Design review of the part built by this model. Coordinates are the model's own, in mm. Face numbers are marked on the shaded views. A direction names the side the tool comes from. Give positions to 0.01 mm unless a question says otherwise; leave off trailing zeros. Loops run counter-clockwise (first coordinate to the right, second up) from the corner with the lowest first, then second, coordinate; pieces in that order, holes last. Notation, with made-up numbers: (-9, -12.75) -> (18, -12.75) arc R25 cw to (18, 17.25) -> close; hole circle Ø6 at (47.5, 20). An arc over 180 degrees is marked (long way). Answer in a Markdown table with one row per item. Add a question column.
(1) Consider section A-A on y = 15. Write out the cut boundary in (x, z), then the cut area to 3 significant figures.
(2) For the marked faces 5, 6, 7, 8 and 9, list the 3-axis set-ups (+Z, -Z, +X, -X, +Y, -Y) from which the entire face can be reached by the end or side of a thin tool; tool diameter is ignored.
(3) For pin 1 (3.5 mm diameter, centred on x = 0, y = 49, fed in from -Z); pin 2 (0.5 mm diameter, centred on y = 49, z = 0.5, fed in from -X); pin 3 (2 mm diameter, centred on x = -4.5, z = -6.5, fed in from +Y); pin 4 (6 mm diameter, centred on x = 0.5, z = -0.5, fed in from -Y), all flat-tipped, find the tip position at first contact; note any pin that passes through.
(4) For line 1 (Y direction, x = 0, z = -0.1); line 2 (Y direction, x = 0.75, z = 3.75); line 3 (Y direction, x = 6.75, z = 4.5), list the stretches that pass through material, from the lowest coordinate up.
(5) Draft analysis for pull direction Y (two halves, no side actions). For the marked faces 1, 2, 3 and 4, state which applies: +Y half, -Y half, draft (parallel to the pull), parting line (faces both ways), or undercut.
(6) Consider section B-B on y = 38.5. Write out the cut boundary in (x, z).
Autodesk Inventor part; units mm, degrees
ref_plane "YZ Plane" through (0, 0, 0) normal (1, 0, 0) x (0, 1, 0)
ref_plane "XZ Plane" through (0, 0, 0) normal (0, 1, 0) x (-1, 0, 0)
ref_plane "XY Plane" through (0, 0, 0) normal (0, 0, 1) x (1, 0, 0)
sketch "Szkic1" plane through (0, 0, 0) normal (0, 1, 0) x (-1, 0, 0)
  circle A0 centre (0, 0) radius 4.5
  dimension "d0" = 9
extrude "Wyciągnięcie proste1" add sketch "Szkic1" along normal blind 2
sketch "Szkic2" plane through (0, 2, 0) normal (0, 1, 0) x (1, 0, 0)
  circle A0 centre (0, 0) radius 2
  dimension "d3" = 4
extrude "Wyciągnięcie proste2" add sketch "Szkic2" along normal blind 30
sketch "Szkic3" plane through (0, 32, 0) normal (0, 1, 0) x (1, 0, 0)
  circle A0 centre (0, 0) radius 6
  dimension "d6" = 12
extrude "Wyciągnięcie proste3" add sketch "Szkic3" along normal blind 5
sketch "Szkic4" plane through (0, 37, 0) normal (0, 1, 0) x (1, 0, 0)
  circle A0 centre (0, 0) radius 8.5
  dimension "d9" = 17
extrude "Wyciągnięcie proste4" add sketch "Szkic4" along normal blind 2
sketch "Szkic5" plane through (0, 39, 0) normal (0, 1, 0) x (1, 0, 0)
  circle A0 centre (0, 0) radius 5
  dimension "d12" = 10
extrude "Wyciągnięcie proste5" add sketch "Szkic5" along normal blind 2.5
sketch "Szkic6" plane through (0, 41.5, 0) normal (0, 1, 0) x (1, 0, 0)
  circle A0 centre (0, 0) radius 2.5
  dimension "d15" = 5
extrude "Wyciągnięcie proste6" add sketch "Szkic6" along normal blind 3
sketch "Szkic7" plane through (0, 44.5, 0) normal (0, 1, 0) x (1, 0, 0)
  line L0 (4.5, -2.5) -> (-4.5, -2.5)
  line L1 (-4.5, -2.5) -> (-4.5, 2.5)
  line L2 (-4.5, 2.5) -> (4.5, 2.5)
  line L3 (4.5, 2.5) -> (4.5, -2.5)
  line L4 (4.5, -2.5) -> (-4.5, 2.5) construction
  line L5 (-4.5, -2.5) -> (4.5, 2.5) construction
  point P0 (0, 0)
  dimension "d18" = 9
  dimension "d19" = 5
extrude "Wyciągnięcie proste7" add sketch "Szkic7" along normal blind 9
fillet "Zaokrąglenie1" radius 4 4 edges at (4.5, 44.5, 0) (4.5, 53.5, 0) (-4.5, 53.5, 0) (-4.5, 44.5, 0)
sketch "Szkic8" plane through (-0.5, 44.5, 2.5) normal (0, 0, 1) x (1, 0, 0)
  line L0 (0, 9) -> (1, 9)
  line L1 (-4, 4) -> (-4, 5)
  circle A0 centre (0.5, 4.5) radius 1.5
  line L2 (0, 0) -> (0.5, 0)
  line L3 (5, 4) -> (5, 5)
  point P0 (0.5, -44.5)
  dimension "d23" = 3
  dimension "d26" = 9
  dimension "d27" = 9
  dimension "d28" = 4.5
  dimension "d29" = 4.5
extrude "Wyciągnięcie proste8" cut sketch "Szkic8" against normal blind 10
fillet "Zaokrąglenie2" radius 1 4 edges at (-8.5, 39, 0) (-5, 39, 0) (-5, 41.5, 0) (-2.5, 41.5, 0)
equation "\"d28\" = 0.5 * d26"
properties part number "Tlok" material "Aluminum 6061"
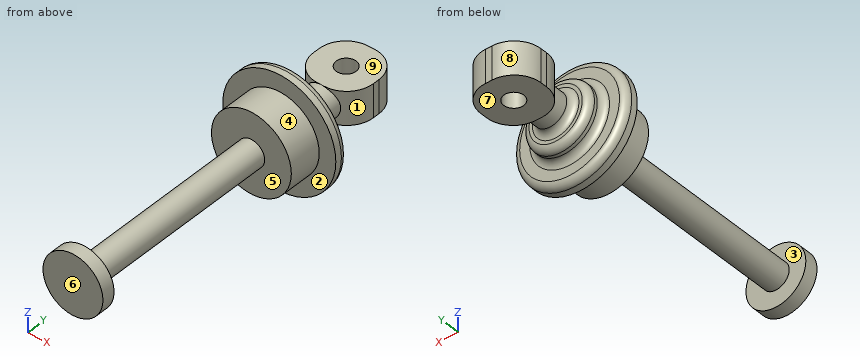
Values follow:
| question | item | result |
|---|---|---|
| 1 | outline | circle Ø4 at (0, 0) |
| 1 | area | 12.6 mm2 |
| 2 | face 5 | none |
| 2 | face 6 | +Z, -Z, +X, -X, -Y |
| 2 | face 7 | -Z, +X, -X, +Y |
| 2 | face 8 | +Z, -Z, -X, +Y |
| 2 | face 9 | +Z, +X, -X, +Y |
| 3 | pin 1 | z = -2.5 |
| 3 | pin 2 | x = -4.5 |
| 3 | pin 3 | y = 39 |
| 3 | pin 4 | y = 0 |
| 4 | line 1 | 0 to 47.5, 50.5 to 53.5 |
| 4 | line 2 | 0 to 2, 32 to 41.5 |
| 4 | line 3 | 37 to 38.79 |
| 5 | face 1 | undercut |
| 5 | face 2 | -Y half |
| 5 | face 3 | undercut |
| 5 | face 4 | draft |
| 6 | outline | circle Ø16.73 at (0, 0) |
